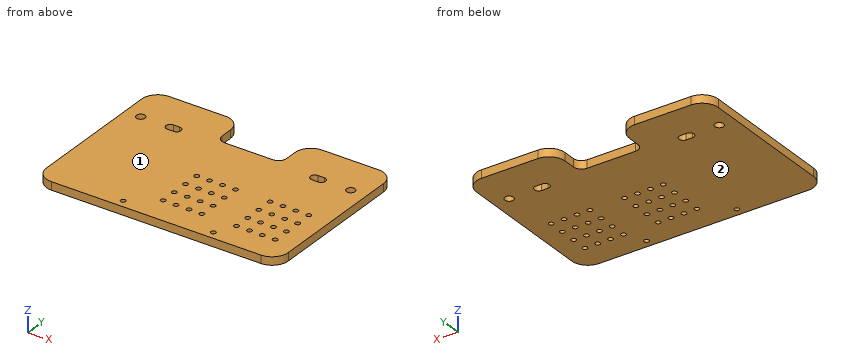
Autodesk Fusion 360 part; units mm, degrees
sketch "草图1" plane through (0, 0, 0) normal (0, 0, 1) x (1, 0, 0)
  line L0 (75, -52.5) -> (-75, -52.5)
  line L1 (-75, -52.5) -> (-75, 52.5)
  line L2 (-75, 52.5) -> (75, 52.5)
  line L3 (75, 52.5) -> (75, -52.5)
  line L4 (75, -52.5) -> (-75, 52.5) construction
  line L5 (-75, -52.5) -> (75, 52.5) construction
  line L6 (-75, 27.5) -> (75, 27.5) construction
  line L7 (0, 52.5) -> (0, 0) construction
  line L8 (-35, 52.5) -> (-35, 27.5) construction
  line L9 (35, 52.5) -> (35, 27.5) construction
  circle A0 centre (-65.15, 27.5) radius 2.65
  circle A1 centre (65.15, 27.5) radius 2.65
  line L10 (-65.15, 30.15) -> (-65.15, 24.85) construction
  line L11 (65.15, 24.85) -> (65.15, 30.15) construction
  line L12 (65.15, 24.85) -> (-65.15, 24.85)
  line L13 (-65.15, 30.15) -> (65.15, 30.15)
  circle A2 centre (-46.85, 27.5) radius 2.65
  circle A3 centre (-42.85, 27.5) radius 2.65
  circle A4 centre (42.85, 27.5) radius 2.65
  circle A5 centre (46.85, 27.5) radius 2.65
  line L14 (-75, -5.5) -> (75, -5.5) construction
  line L15 (-75, -35.5) -> (75, -35.5) construction
  line L16 (-75, -47.5) -> (75, -47.5) construction
  circle A6 centre (-24, -47.5) radius 1.525
  circle A7 centre (32, -47.5) radius 1.525
  line L17 (-75, -25.5) -> (75, -25.5) construction
  line L18 (-75, -15.5) -> (75, -15.5) construction
  line L19 (62, -35.5) -> (62, -5.5) construction
  line L20 (-7.5, -35.5) -> (-7.5, -5.5) construction
  line L21 (0.5, -35.5) -> (0.5, -5.5) construction
  line L22 (8.5, -35.5) -> (8.5, -5.5) construction
  line L23 (16.5, -35.5) -> (16.5, -5.5) construction
  line L24 (38, -35.5) -> (38, -5.5) construction
  line L25 (46, -35.5) -> (46, -5.5) construction
  line L26 (54, -35.5) -> (54, -5.5) construction
  circle A8 centre (62, -5.5) radius 1.5
  circle A9 centre (62, -15.5) radius 1.5
  circle A10 centre (62, -25.5) radius 1.5
  circle A11 centre (62, -35.5) radius 1.5
  circle A12 centre (54, -5.5) radius 1.5
  circle A13 centre (54, -15.5) radius 1.5
  circle A14 centre (54, -25.5) radius 1.5
  circle A15 centre (54, -35.5) radius 1.5
  circle A16 centre (46, -5.5) radius 1.5
  circle A17 centre (46, -15.5) radius 1.5
  circle A18 centre (46, -25.5) radius 1.5
  circle A19 centre (38, -25.5) radius 1.5
  circle A20 centre (38, -5.5) radius 1.5
  circle A21 centre (38, -15.5) radius 1.5
  circle A22 centre (38, -35.5) radius 1.5
  circle A23 centre (46, -35.5) radius 1.5
  circle A24 centre (16.5, -5.5) radius 1.5
  circle A25 centre (8.5, -5.5) radius 1.5
  circle A26 centre (0.5, -5.5) radius 1.5
  circle A27 centre (-7.5, -5.5) radius 1.5
  circle A28 centre (16.5, -15.5) radius 1.5
  circle A29 centre (8.5, -15.5) radius 1.5
  circle A30 centre (0.5, -15.5) radius 1.5
  circle A31 centre (-7.5, -15.5) radius 1.5
  circle A32 centre (-7.5, -25.5) radius 1.5
  circle A33 centre (0.5, -25.5) radius 1.5
  circle A34 centre (8.5, -25.5) radius 1.5
  circle A35 centre (16.5, -25.5) radius 1.5
  circle A36 centre (16.5, -35.5) radius 1.5
  circle A37 centre (8.5, -35.5) radius 1.5
  circle A38 centre (0.5, -35.5) radius 1.5
  circle A39 centre (-7.5, -35.5) radius 1.5
  line L27 (-20, 52.5) -> (-20, 30.15)
  line L28 (20, 52.5) -> (20, 30.15)
  point P0 (-65.15, 27.5)
  point P1 (65.15, 27.5)
  point P2 (-44.85, 27.5)
  point P3 (44.85, 27.5)
  point P4 (0, 27.5)
  point P5 (-46.85, 27.5)
  point P6 (-42.85, 27.5)
  point P7 (42.85, 27.5)
  point P8 (46.85, 27.5)
  point P9 (32, -47.5)
  point P10 (-24, -47.5)
  point P11 (0.5, -35.5)
  point P12 (8.5, -35.5)
  point P13 (16.5, -35.5)
  point P14 (-7.5, -25.5)
  point P15 (-7.5, -5.5)
  point P16 (-7.5, -35.5)
  point P17 (-7.5, -15.5)
  point P18 (-7.5, -25.5)
  point P19 (62, -35.5)
  point P20 (62, -25.5)
  point P21 (62, -15.5)
  point P22 (62, -5.5)
  point P23 (54, -35.5)
  point P24 (46, -35.5)
  point P25 (38, -35.5)
  point P26 (0.5, -25.5)
  point P27 (0.5, -15.5)
  point P28 (0.5, -5.5)
  point P29 (8.5, -25.5)
  point P30 (8.5, -15.5)
  point P31 (8.5, -5.5)
  point P32 (16.5, -25.5)
  point P33 (16.5, -15.5)
  point P34 (16.5, -5.5)
  point P35 (38, -25.5)
  point P36 (38, -15.5)
  point P37 (38, -5.5)
  point P38 (46, -25.5)
  point P39 (46, -15.5)
  point P40 (46, -5.5)
  point P41 (54, -25.5)
  point P42 (54, -15.5)
  point P43 (54, -5.5)
  dimension "d1" = 150
  dimension "d2" = 105
  dimension "d3" = 25
  dimension "d4" = 20.3
  dimension "d5" = 20.3
  dimension "d6" = 9.85
  dimension "d7" = 44.85
  dimension "d8" = 9.85
  dimension "d9" = 44.85
  dimension "d10" = 40
  dimension "d11" = 40
  dimension "d12" = 70
  dimension "d13" = 5.3
  dimension "d14" = 5.3
  dimension "d15" = 2
  dimension "d16" = 2
  dimension "d17" = 2
  dimension "d18" = 2
  dimension "d20" = 30
  dimension "d24" = 56
  dimension "d25" = 3.05
  dimension "d26" = 3.05
  dimension "d27" = 10
  dimension "d28" = 10
  dimension "d29" = 10
  dimension "d30" = 13
  dimension "d35" = 8
  dimension "d36" = 16
  dimension "d37" = 24
  dimension "d38" = 3
  dimension "d39" = 3
  dimension "d40" = 3
  dimension "d41" = 3
  dimension "d42" = 3
  dimension "d43" = 3
  dimension "d44" = 3
  dimension "d45" = 3
  dimension "d46" = 3
  dimension "d47" = 3
  dimension "d48" = 3
  dimension "d49" = 3
  dimension "d50" = 3
  dimension "d51" = 3
  dimension "d52" = 3
  dimension "d53" = 3
  dimension "d54" = 3
  dimension "d55" = 3
  dimension "d56" = 3
  dimension "d57" = 3
  dimension "d58" = 3
  dimension "d59" = 3
  dimension "d60" = 3
  dimension "d61" = 3
  dimension "d62" = 3
  dimension "d63" = 3
  dimension "d64" = 3
  dimension "d65" = 3
  dimension "d66" = 3
  dimension "d67" = 3
  dimension "d68" = 3
  dimension "d69" = 3
  dimension "d72" = 21.5
  dimension "d73" = 21.5
  dimension "d74" = 8
  dimension "d75" = 8
  dimension "d76" = 8
  dimension "d77" = 20
  dimension "d84" = 51
  dimension "d87" = 5
  dimension "d88" = 12
extrude "拉伸4" add sketch "草图1" along normal blind 5 contours L0 L1 L2 L3 A0 A1 L12 L13 L27 L28 | L12 L13 A3 A4 | A1 L12 L13 A5 | A0 L12 L13 A2
fillet "圆角3" radius 10 6 edges at (-75, 52.5, 2.5) (-75, -52.5, 2.5) (75, -52.5, 2.5) (-20, 52.5, 2.5) (75, 52.5, 2.5) (20, 52.5, 2.5)
fillet "圆角4" radius 5 2 edges at (-20, 30.15, 2.5) (20, 30.15, 2.5)
sketch "草图2" plane through (0, 0, 5) normal (0, 0, 1) x (-1, 0, 0)
  arc A0 (-30, -52.5) -> (-20, -42.5) centre (-30, -42.5) ccw
  line L0 (-20, -42.5) -> (-20, -35.15)
  arc A1 (-15, -30.15) -> (-20, -35.15) centre (-15, -35.15) ccw
  line L1 (-15, -30.15) -> (15, -30.15)
  arc A2 (20, -35.15) -> (15, -30.15) centre (15, -35.15) ccw
  line L2 (20, -35.15) -> (20, -42.5)
  arc A3 (20, -42.5) -> (30, -52.5) centre (30, -42.5) ccw
  line L3 (30, -52.5) -> (65, -52.5)
  arc A4 (65, -52.5) -> (75, -42.5) centre (65, -42.5) ccw
  line L4 (75, -42.5) -> (75, 42.5)
  arc A5 (75, 42.5) -> (65, 52.5) centre (65, 42.5) ccw
  line L5 (65, 52.5) -> (-65, 52.5)
  arc A6 (-65, 52.5) -> (-75, 42.5) centre (-65, 42.5) ccw
  line L6 (-75, 42.5) -> (-75, -42.5)
  arc A7 (-75, -42.5) -> (-65, -52.5) centre (-65, -42.5) ccw
  line L7 (-65, -52.5) -> (-30, -52.5)
  circle A8 centre (7.5, 15.5) radius 1.5
  circle A9 centre (7.5, 25.5) radius 1.5
  circle A10 centre (-8.5, 25.5) radius 1.5
  circle A11 centre (-0.5, 25.5) radius 1.5
  arc A12 (46.85, -30.15) -> (46.85, -24.85) centre (46.85, -27.5) ccw
  line L8 (46.85, -30.15) -> (42.85, -30.15)
  arc A13 (42.85, -24.85) -> (42.85, -30.15) centre (42.85, -27.5) ccw
  line L9 (42.85, -24.85) -> (46.85, -24.85)
  circle A14 centre (65.15, -27.5) radius 2.65
  arc A15 (-42.85, -30.15) -> (-42.85, -24.85) centre (-42.85, -27.5) ccw
  line L10 (-42.85, -30.15) -> (-46.85, -30.15)
  arc A16 (-46.85, -24.85) -> (-46.85, -30.15) centre (-46.85, -27.5) ccw
  line L11 (-46.85, -24.85) -> (-42.85, -24.85)
  circle A17 centre (-0.5, 35.5) radius 1.5
  circle A18 centre (-16.5, 25.5) radius 1.5
  circle A19 centre (-16.5, 35.5) radius 1.5
  circle A20 centre (-8.5, 35.5) radius 1.5
  circle A21 centre (-65.15, -27.5) radius 2.65
  circle A22 centre (7.5, 35.5) radius 1.5
  circle A23 centre (-0.5, 15.5) radius 1.5
  circle A24 centre (-8.5, 15.5) radius 1.5
  circle A25 centre (-16.5, 15.5) radius 1.5
  circle A26 centre (7.5, 5.5) radius 1.5
  circle A27 centre (-0.5, 5.5) radius 1.5
  circle A28 centre (-8.5, 5.5) radius 1.5
  circle A29 centre (-16.5, 5.5) radius 1.5
  circle A30 centre (-46, 35.5) radius 1.5
  circle A31 centre (-38, 35.5) radius 1.5
  circle A32 centre (-38, 15.5) radius 1.5
  circle A33 centre (-38, 5.5) radius 1.5
  circle A34 centre (-38, 25.5) radius 1.5
  circle A35 centre (-46, 25.5) radius 1.5
  circle A36 centre (-46, 15.5) radius 1.5
  circle A37 centre (-46, 5.5) radius 1.5
  circle A38 centre (-54, 35.5) radius 1.5
  circle A39 centre (-54, 25.5) radius 1.5
  circle A40 centre (-54, 15.5) radius 1.5
  circle A41 centre (-54, 5.5) radius 1.5
  circle A42 centre (-62, 35.5) radius 1.5
  circle A43 centre (-62, 25.5) radius 1.5
  circle A44 centre (-62, 15.5) radius 1.5
  circle A45 centre (-62, 5.5) radius 1.5
  circle A46 centre (-32, 47.5) radius 1.525
  circle A47 centre (24, 47.5) radius 1.525
  circle A48 centre (-32, 47.5) radius 1.525
  circle A49 centre (24, 47.5) radius 1.525
  circle A50 centre (7.5, 35.5) radius 1.5
  circle A51 centre (-0.5, 35.5) radius 1.5
  circle A52 centre (-8.5, 35.5) radius 1.5
  circle A53 centre (-16.5, 35.5) radius 1.5
  circle A54 centre (-38, 35.5) radius 1.5
  circle A55 centre (-46, 35.5) radius 1.5
  circle A56 centre (-54, 35.5) radius 1.5
  circle A57 centre (-62, 35.5) radius 1.5
  circle A58 centre (-62, 25.5) radius 1.5
  circle A59 centre (-54, 25.5) radius 1.5
  circle A60 centre (-46, 25.5) radius 1.5
  circle A61 centre (-38, 25.5) radius 1.5
  circle A62 centre (-16.5, 25.5) radius 1.5
  circle A63 centre (-8.5, 25.5) radius 1.5
  circle A64 centre (-0.5, 25.5) radius 1.5
  circle A65 centre (7.5, 25.5) radius 1.5
  circle A66 centre (7.5, 15.5) radius 1.5
  circle A67 centre (-0.5, 15.5) radius 1.5
  circle A68 centre (-8.5, 15.5) radius 1.5
  circle A69 centre (-16.5, 15.5) radius 1.5
  circle A70 centre (-38, 15.5) radius 1.5
  circle A71 centre (-46, 15.5) radius 1.5
  circle A72 centre (-54, 15.5) radius 1.5
  circle A73 centre (-62, 15.5) radius 1.5
  circle A74 centre (-62, 5.5) radius 1.5
  circle A75 centre (-54, 5.5) radius 1.5
  circle A76 centre (-46, 5.5) radius 1.5
  circle A77 centre (-38, 5.5) radius 1.5
  circle A78 centre (-16.5, 5.5) radius 1.5
  circle A79 centre (-8.5, 5.5) radius 1.5
  circle A80 centre (-0.5, 5.5) radius 1.5
  circle A81 centre (7.5, 5.5) radius 1.5
  circle A82 centre (65.15, -27.5) radius 2.65
  circle A83 centre (-65.15, -27.5) radius 2.65
  line L12 (-46.85, -24.85) -> (-42.85, -24.85)
  line L13 (-46.85, -30.15) -> (-42.85, -30.15)
  arc A84 (-46.85, -24.85) -> (-46.85, -30.15) centre (-46.85, -27.5) ccw
  arc A85 (-42.85, -30.15) -> (-42.85, -24.85) centre (-42.85, -27.5) ccw
  arc A86 (42.85, -24.85) -> (42.85, -30.15) centre (42.85, -27.5) ccw
  arc A87 (46.85, -30.15) -> (46.85, -24.85) centre (46.85, -27.5) ccw
  line L14 (42.85, -24.85) -> (46.85, -24.85)
  line L15 (42.85, -30.15) -> (46.85, -30.15)
  line L16 (-65, -52.5) -> (-30, -52.5)
  line L17 (-20, -42.5) -> (-20, -35.15)
  line L18 (20, -35.15) -> (20, -42.5)
  line L19 (15, -30.15) -> (-15, -30.15)
  line L20 (30, -52.5) -> (65, -52.5)
  line L21 (-75, -42.5) -> (-75, 42.5)
  line L22 (-65, 52.5) -> (65, 52.5)
  line L23 (75, 42.5) -> (75, -42.5)
  arc A88 (-65, 52.5) -> (-75, 42.5) centre (-65, 42.5) ccw
  arc A89 (75, 42.5) -> (65, 52.5) centre (65, 42.5) ccw
  arc A90 (65, -52.5) -> (75, -42.5) centre (65, -42.5) ccw
  arc A91 (20, -42.5) -> (30, -52.5) centre (30, -42.5) ccw
  arc A92 (20, -35.15) -> (15, -30.15) centre (15, -35.15) ccw
  arc A93 (-15, -30.15) -> (-20, -35.15) centre (-15, -35.15) ccw
  arc A94 (-30, -52.5) -> (-20, -42.5) centre (-30, -42.5) ccw
  arc A95 (-75, -42.5) -> (-65, -52.5) centre (-65, -42.5) ccw
  dimension "d95" = 21.5
extrude "拉伸3" [suppressed]
extrude "拉伸2" [suppressed]
fillet "圆角1" [suppressed]
fillet "圆角2" [suppressed]
extrude "拉伸1" [suppressed]
Input: part model. Units: mm. Frame: model coordinates. Face numbers are marked on the shaded views. Coordinates: 2 decimals unless noted, no trailing zeros. Loops run counter-clockwise (first coordinate to the right, second up) from the corner with the lowest first, then second, coordinate; pieces in that order, holes last. Notation, with made-up numbers: (-13, -29) - (-6, -29) arc R17 ccw to (-6, -20) - close; hole circle Ø11 at (26, 23). An arc over 180 degrees is marked (long way). Answer in a Markdown table with one row per item. Add a question column.
Item 1: Mould query, pull axis Z, two halves, no side actions, for the marked faces 1 and 2. Classes: released by +Z, released by -Z, zero draft, split by the parting line, or undercut.
Item 2: Line query: line 1 along Y through (x, z) = (46, 4.05); line 2 along X through (y, z) = (27.5, 2.7); line 3 along Y through (x, z) = (0.5, 4). Output: solid intervals per line, ascending. Write a range as [from, to].
Item 3: Contact query for flat-ended pins moving along their axis: P1, Ø6, axis at x = -65.15, y = 27.5, coming from the +Z side; P2, Ø1.8, axis at x = 38, y = -25.5, coming from the -Z side. Output: stop coordinate, or through.
Item 4: Section query A-A on x = 8.5. Return the cut outline in (y, z).
Item 5: Section query C-C on y = -47.5. Return the cut outline in (x, z) (3 decimals), then the cut area to 3 significant figures.
Item 6: Section query B-B on x = -24. Return the cut outline in (y, z) (3 decimals).
Item 7: Section query D-D on z = 2.4. State how many separate pieces and enclosed holes the cut face has, then the cut area to 3 significant figures.
Recorded:
| question | item | result |
|---|---|---|
| 1 | face 1 | released by +Z |
| 1 | face 2 | released by -Z |
| 2 | line 1 | [-52.5, -37], [-34, -27], [-24, -17], [-14, -7], [-4, 24.85], [30.15, 52.5] |
| 2 | line 2 | [-75, -67.8], [-62.5, -49.5], [-40.2, 40.2], [49.5, 62.5], [67.8, 75] |
| 2 | line 3 | [-52.5, -37], [-34, -27], [-24, -17], [-14, -7], [-4, 30.15] |
| 3 | P1 | z = 5 |
| 3 | P2 | through |
| 4 | outline | (-52.5, 0) - (-37, 0) - (-37, 5) - (-52.5, 5) - close; (-34, 0) - (-27, 0) - (-27, 5) - (-34, 5) - close; (-24, 0) - (-17, 0) - (-17, 5) - (-24, 5) - close; (-14, 0) - (-7, 0) - (-7, 5) - (-14, 5) - close; (-4, 0) - (30.15, 0) - (30.15, 5) - (-4, 5) - close |
| 5 | outline | (-73.66, 0) - (-25.525, 0) - (-25.525, 5) - (-73.66, 5) - close; (-22.475, 0) - (30.475, 0) - (30.475, 5) - (-22.475, 5) - close; (33.525, 0) - (73.66, 0) - (73.66, 5) - (33.525, 5) - close |
| 5 | area | 706 mm^2 |
| 6 | outline | (-52.5, 0) - (-49.025, 0) - (-49.025, 5) - (-52.5, 5) - close; (-45.975, 0) - (50.5, 0) - (50.5, 5) - (-45.975, 5) - close |
| 7 | separate pieces | 1 |
| 7 | enclosed holes | 38 |
| 7 | area | 14,400 mm^2 |
